Part print with two shaded views. Sizes in mm from the minimum x, y, z corner. A direction names the side the tool comes from. Round coordinates to 2 decimals unless told otherwise and drop trailing zeros. Write each loop counter-clockwise with the first axis right and the second up, starting at its lowest first coordinate (ties: lowest second). Pieces come first, ordered by that corner, then holes. Notation, with made-up numbers: (10.5, 22.25) -> (24.5, 22.25) arc R30 ccw to (24.5, 59.25) -> close; hole circle Ø5 at (41.5, 83). An arc over 180 degrees is marked (long way). Return JSON: item names as keys, results as strings.
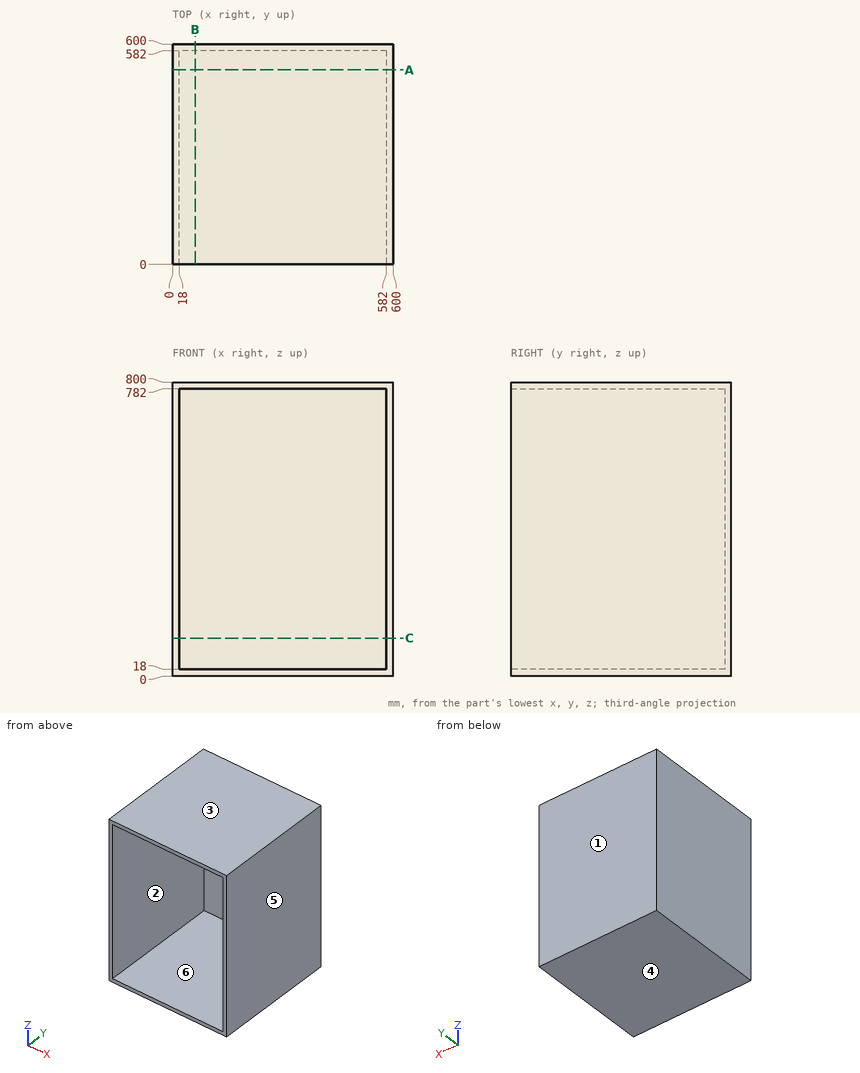
Q1. Saw through at A-A on y = 529.5. List the corners of the cut face in (x, z), then the cut area to 3 significant figures.
Verdict:
{"outline": "(0, 0) -> (600, 0) -> (600, 800) -> (0, 800) -> close; hole (18, 18) -> (582, 18) -> (582, 782) -> (18, 782) -> close", "area": "49,100 mm²"}
Q2. Pin check, flat tip, straight feed: pin 1 Ø5 at (x, z) = (480, 590.5) entering from -Y. Stop position of the tip, or through.
Verdict:
{"pin 1": "stops at y = 582"}
Q3. Two-plate mould, pull along Z, no slides. Class the marked faces 1, 2, 3 and 4: +Z half, -Z half, draft (parallel to the pull), parting line (faces both ways), or undercut.
Verdict:
{"face 1": "draft", "face 2": "undercut", "face 3": "+Z half", "face 4": "-Z half"}
Q4. 3-axis set-ups, long thin cutter, end or side, ignore diameter. For the marked faces 5 and 6: which of +Z, -Z, +X, -X, +Y, -Y reach the whole face in a straight line?
Verdict:
{"face 5": "+Z, -Z, +X, +Y, -Y", "face 6": "-Y"}
Q5. Saw through at C-C on z = 103. List the corners of the cut face in (x, y), then the cut area to 3 significant figures.
Verdict:
{"outline": "(0, 0) -> (18, 0) -> (18, 582) -> (582, 582) -> (582, 0) -> (600, 0) -> (600, 600) -> (0, 600) -> close", "area": "31,800 mm²"}
Q6. Saw through at B-B on x = 61. List the corners of the cut face in (y, z), then the cut area to 3 significant figures.
Verdict:
{"outline": "(0, 0) -> (600, 0) -> (600, 800) -> (0, 800) -> (0, 782) -> (582, 782) -> (582, 18) -> (0, 18) -> close", "area": "35,400 mm²"}
Q7. Wall check: L1, parallel to X at y = 373.5, z = 362; L2, parallel to Z at x = 332, y = 326.5; L3, parallel to Y at x = 575.5, z = 153.5. Give the ranges that are in metal, low to high.
Verdict:
{"L1": "x = 0 to 18, 582 to 600", "L2": "z = 0 to 18, 782 to 800", "L3": "y = 582 to 600"}
